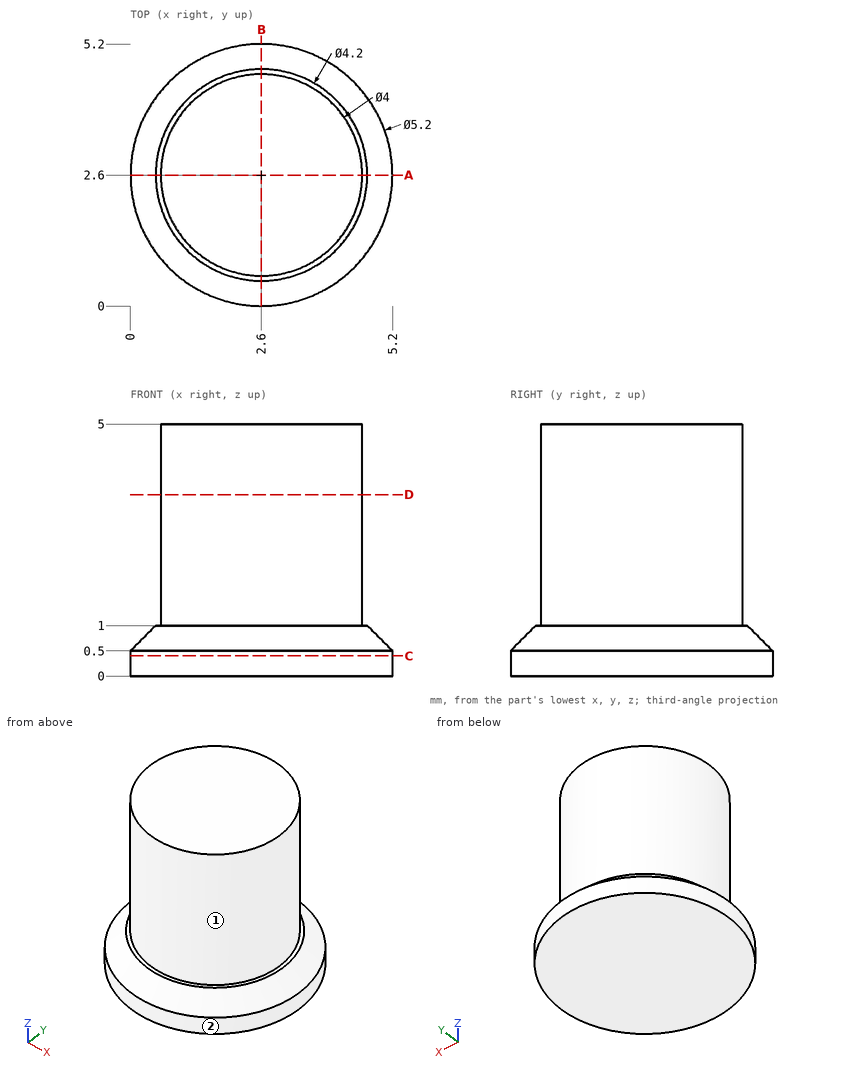
Drawing for the job (mm, zero at the part's lowest x, y, z). A direction names the side the tool comes from. Round coordinates to 2 decimals unless told otherwise and drop trailing zeros. Write each loop counter-clockwise with the first axis right and the second up, starting at its lowest first coordinate (ties: lowest second). Pieces come first, ordered by that corner, then holes.
Item 1: Drill centre lines: L1, parallel to X at y = 2.55, z = 3.05; L2, parallel to Y at x = 2.3, z = 1.15; L3, parallel to Y at x = 3.55, z = 1.75. Where is each one in solid material? Low to high.
Filled in:
L1: x = 0.6 to 4.6
L2: y = 0.62 to 4.58
L3: y = 0.84 to 4.36
Item 2: Band-saw the part on A-A on y = 2.6. Write the cut outline in (x, z).
Filled in:
outline: (0, 0) - (5.2, 0) - (5.2, 0.5) - (4.7, 1) - (4.6, 1) - (4.6, 5) - (0.6, 5) - (0.6, 1) - (0.5, 1) - (0, 0.5) - close
Item 3: Tool access for the marked faces 1 and 2: list every direction of +Z, -Z, +X, -X, +Y, -Y with a clear straight run to the whole face (end or side of a thin tool).
Filled in:
face 1: +Z
face 2: +Z, -Z
Item 4: Band-saw the part on D-D on z = 3.6. Write the cut outline in (x, y).
Filled in:
outline: circle Ø4 at (2.6, 2.6)
Item 5: Band-saw the part on C-C on z = 0.4. Write the cut outline in (x, y), then the cut area to 3 significant figures.
Filled in:
outline: circle Ø5.2 at (2.6, 2.6)
area: 21.2 mm2
